Work out the finished part from the listing and answer in its coordinate system (mm). A direction names the side the tool comes from. Coordinates: 2 decimals unless noted, no trailing zeros. Order: outer loops, then holes, each group sorted by start corner. A loop starts at its lowest first (then second) coordinate and runs counter-clockwise, first axis right, second up. Notation, with made-up numbers: M 51,55.25 L 91,55.25 A13 ccw 91,64.25 Z; hole C 46,21.5 d2. An arc over 180 degrees is marked long. Answer in a Markdown table with one row per item. Add a question column.
Item 1: The part is cut by section A-A (y = 1.75). Write down the section's boundary in (x, z), then the cut area to 3 significant figures.
Item 2: The part is cut by section B-B (y = 12). Write down the section's boundary in (x, z).
Item 3: Consider line 1 (X direction, y = 2, z = 6); line 2 (X direction, y = 11, z = 5); line 3 (X direction, y = 14.75, z = 6). Determine where each line is inside the solid, lowest interval first. Write a range as from..to.
Item 4: Which of the six approach directions +Z, -Z, +X, -X, +Y, -Y give full straight-line access (tool end or side, diameter ignored) to faces 1 (the face through (0, 18, 2.25)), 2 (the face through (12.785, 9.486, 4.644)), 3 (the face through (10, 17.5, 6))?
Item 5: Flat-ended cylindrical pins translate along their axes: pin 1 Ø3 at (x, z) = (0, -12) entering from -Y; pin 2 Ø4 at (x, y) = (2.5, 17) entering from +Z; pin 3 Ø4 at (x, z) = (-5, 0.5) entering from -Y. Find the tip coordinate at first contact, or state that the pin passes through.
from build123d import *

# Parameters (mm, degrees)
SKETCH1_R                 = 17
SKETCH1_R_2               = 1.6000000000000005
SKETCH1_R_3               = 1.6000000000000019
SKETCH1_R_4               = 1.5999999999999999
BOSS_EXTRUDE1_DEPTH       = 6.500000000000001
SKETCH2_R                 = 17
SKETCH2_R_2               = 3.4999999999999996
SKETCH2_R_3               = 1.6000000000000012
SKETCH2_R_4               = 1.6000000000000019
SKETCH2_R_5               = 1.5999999999999963
BOSS_EXTRUDE2_DEPTH       = 2
SKETCH3_R                 = 17
SKETCH3_R_2               = 1.2
BOSS_EXTRUDE3_DEPTH       = 2
SKETCH9_R                 = 17
SKETCH9_R_2               = 1.2
SKETCH9_R_3               = 1.5999999999999963
SKETCH9_R_4               = 1.6000000000000012
SKETCH9_R_5               = 1.6000000000000019
BOSS_EXTRUDE6_DEPTH       = 2
BOSS_EXTRUDE4_OUTLINE_R   = 17
BOSS_EXTRUDE4_OUTLINE_R_2 = 1.6
BOSS_EXTRUDE4_DEPTH       = 5
SKETCH10_R                = 17
BOSS_EXTRUDE7_DEPTH       = 4.500000000000001
CHAMFER1_SIZE             = 1.154700538
CHAMFER1_SIZE_2           = 2


# Read off the part's stored shape, not the designer's step: Boss-Extrude4
with BuildPart() as part:
    # Sketch1 → Boss-Extrude1 (new body)
    with BuildSketch(Plane(origin=(0, 0, 0), x_dir=(1, 0, 0), z_dir=(0, 1, 0))):
        with Locations(Location((0, 0, 0), (0, 0, 270))):
            Circle(SKETCH1_R)
        with Locations(Location((0, 12, 0), (0, 0, 270))):
            Circle(SKETCH1_R_2, mode=Mode.SUBTRACT)
        with Locations(Location((10.392304845413268, -5.999999999999997, 0), (0, 0, 270))):
            Circle(SKETCH1_R_3, mode=Mode.SUBTRACT)
        with Locations(Location((-10.39230484541326, -6.000000000000005, 0), (0, 0, 270))):
            Circle(SKETCH1_R_4, mode=Mode.SUBTRACT)
        Polygon((4.04145188432738, -6.999999999999999), (8.082903768654761, -8.7e-16), (4.041451884327381, 6.999999999999999), (-4.041451884327381, 6.999999999999999), (-8.082903768654761, -8.7e-16), (-4.04145188432738, -6.999999999999999), align=None, mode=Mode.SUBTRACT)
    extrude(amount=BOSS_EXTRUDE1_DEPTH)

    # Sketch2 → Boss-Extrude2 (add)
    with BuildSketch(Plane(origin=(0, 6.500000000000001, 0), x_dir=(1, 0, 0), z_dir=(0, 1, 0))):
        with Locations(Location((0, 0, 0), (0, 0, 270))):
            Circle(SKETCH2_R)
        with Locations(Location((0, 0, 0), (0, 0, 270))):
            Circle(SKETCH2_R_2, mode=Mode.SUBTRACT)
        with Locations(Location((0, 12, 0), (0, 0, 270))):
            Circle(SKETCH2_R_3, mode=Mode.SUBTRACT)
        with Locations(Location((10.392304845413268, -5.999999999999997, 0), (0, 0, 270))):
            Circle(SKETCH2_R_4, mode=Mode.SUBTRACT)
        with Locations(Location((-10.39230484541326, -6.000000000000005, 0), (0, 0, 270))):
            Circle(SKETCH2_R_5, mode=Mode.SUBTRACT)
    extrude(amount=BOSS_EXTRUDE2_DEPTH)

    # Sketch3 → Boss-Extrude3 (add)
    with BuildSketch(Plane(origin=(0, 8.5, 0), x_dir=(1, 0, 0), z_dir=(0, 1, 0))):
        with Locations(Location((0, 0, 0), (0, 0, 270))):
            Circle(SKETCH3_R)
        with Locations(Location((0, 0, 0), (0, 0, 270))):
            Circle(SKETCH3_R_2, mode=Mode.SUBTRACT)
        Polygon((3.175426480542944, 11.999999999999996), (1.5877132402714735, 14.75), (-1.5877132402714682, 14.75), (-3.1754264805429417, 11.999999999999995), (-1.5877132402714735, 9.249999999999998), (1.5877132402714729, 9.249999999999998), align=None, mode=Mode.SUBTRACT)
        Polygon((-8.804591605141788, -8.750000000000009), (-7.216878364870316, -6.0000000000000036), (-8.80459160514179, -3.2500000000000013), (-11.980018085684733, -3.250000000000002), (-13.567731325956206, -6.000000000000007), (-11.980018085684732, -8.750000000000009), align=None, mode=Mode.SUBTRACT)
        Polygon((8.804591605141793, -8.75), (11.980018085684742, -8.75), (13.567731325956213, -5.999999999999997), (11.98001808568474, -3.2499999999999925), (8.804591605141791, -3.249999999999992), (7.216878364870319, -5.999999999999996), align=None, mode=Mode.SUBTRACT)
    extrude(amount=BOSS_EXTRUDE3_DEPTH)

    # Sketch9 → Boss-Extrude6 (add)
    with BuildSketch(Plane(origin=(0, 10.5, 0), x_dir=(1, 0, 0), z_dir=(0, 1, 0))):
        with Locations(Location((0, 0, 0), (0, 0, 270))):
            Circle(SKETCH9_R)
        with Locations(Location((0, 0, 0), (0, 0, 270))):
            Circle(SKETCH9_R_2, mode=Mode.SUBTRACT)
        with Locations(Location((-10.39230484541326, -6.000000000000005, 0), (0, 0, 270))):
            Circle(SKETCH9_R_3, mode=Mode.SUBTRACT)
        with Locations(Location((0, 12, 0), (0, 0, 270))):
            Circle(SKETCH9_R_4, mode=Mode.SUBTRACT)
        with Locations(Location((10.392304845413268, -5.999999999999997, 0), (0, 0, 270))):
            Circle(SKETCH9_R_5, mode=Mode.SUBTRACT)
    extrude(amount=BOSS_EXTRUDE6_DEPTH)

    # Boss-Extrude4 outline → Boss-Extrude4 (add)
    with BuildSketch(Plane(origin=(0, 12.5, 0), x_dir=(1, 0, 0), z_dir=(0, 1, 0))):
        Circle(BOSS_EXTRUDE4_OUTLINE_R)
        with Locations((-10.392304845, -6)):
            Circle(BOSS_EXTRUDE4_OUTLINE_R_2, mode=Mode.SUBTRACT)
        with Locations((10.392304845, -6)):
            Circle(BOSS_EXTRUDE4_OUTLINE_R_2, mode=Mode.SUBTRACT)
        with BuildLine():
            Line((-2.34520788, 2.25), (2.34520788, 2.25))
            ThreePointArc((2.34520788, 2.25), (3.25, 0), (2.34520788, -2.25))
            Line((2.34520788, -2.25), (-2.34520788, -2.25))
            ThreePointArc((-2.34520788, -2.25), (-3.25, 0), (-2.34520788, 2.25))
        make_face(mode=Mode.SUBTRACT)
        with Locations((0, 12)):
            Circle(BOSS_EXTRUDE4_OUTLINE_R_2, mode=Mode.SUBTRACT)
    extrude(amount=BOSS_EXTRUDE4_DEPTH)

    # Sketch10 → Boss-Extrude7 (add)
    with BuildSketch(Plane(origin=(0, 17.5, 0), x_dir=(1, 0, 0), z_dir=(0, 1, 0))):
        with Locations(Location((0, 0, 0), (0, 0, 270))):
            Circle(SKETCH10_R)
        with BuildLine():
            Line((-2.345207879911715, -2.2500000000000004), (2.345207879911715, -2.2500000000000004))
            ThreePointArc((2.345207879911715, -2.2500000000000004), (3.2500000000000004, 0), (2.345207879911715, 2.2500000000000004))
            Line((2.345207879911715, 2.2500000000000004), (-2.345207879911715, 2.2500000000000004))
            ThreePointArc((-2.345207879911715, 2.2500000000000004), (-3.2500000000000004, 4e-16), (-2.345207879911715, -2.2500000000000004))
        make_face(mode=Mode.SUBTRACT)
    extrude(amount=BOSS_EXTRUDE7_DEPTH)

    # Sketch5 → Cut-Revolve2 (revolve, cut)
    with BuildSketch(Plane(origin=(0, 0, 0), x_dir=(0, 0, -1), z_dir=(1, 0, 0)), mode=Mode.PRIVATE) as cut_revolve2_sk:
        Polygon((-17, 18.535898384862204), (-15.000000000000002, 22), (-17, 22.000000000000004), align=None)
    revolve(cut_revolve2_sk.sketch.rotate(Axis((0, 0, 0), (0, 1, 0)), 180), axis=Axis((0, 0, 0), (0, 1, 0)), mode=Mode.SUBTRACT)

    # Chamfer1
    # the kernel refuses this chamfer: 2, 1.154700538 mm, written as the material it adds along each edge
    with BuildSketch(Plane(origin=(-2.2883428e-10, 12.5, 0), x_dir=(-0.7079171545098687, 0, -0.706295478076032), z_dir=(-0.706295478076032, 0, 0.7079171545098687))) as chamfer1_piece_1:
        Polygon((3.2500000002288263 - CHAMFER1_SIZE, 0), (3.2500000002288343, -CHAMFER1_SIZE_2), (3.2500000002288263, 0), align=None)
    revolve(axis=Axis((-2.2883428e-10, 12.5, 0), (0, -1, 0)), revolution_arc=270.1314019865591)
    with BuildSketch(Plane(origin=(-7.519379389291984, 12.5, -2.2500000000000004), x_dir=(0, 0.9998132206222079, -0.01932676561270072), z_dir=(1, 0, 0))) as chamfer1_piece_2_section:
        Polygon((CHAMFER1_SIZE_2 * 0.999813220622, CHAMFER1_SIZE_2 * 0.0193267656127), (-CHAMFER1_SIZE * 0.019326765619, CHAMFER1_SIZE * 0.999813220951), (0, 0), align=None)
    chamfer1_piece_2 = extrude(amount=15.038758778583968, mode=Mode.PRIVATE)
    chamfer1_piece_2 = chamfer1_piece_2 - Plane(origin=(0, 13.182227685151497, 0), x_dir=(-1.8e-16, 0, 1), z_dir=(0, -1, 0)) * Cylinder(1.2, 39, mode=Mode.PRIVATE)
    add(chamfer1_piece_2)
    with BuildSketch(Plane(origin=(2.2883428e-10, 12.5, 0), x_dir=(0.7079171545098687, 0, 0.706295478076032), z_dir=(0.706295478076032, 0, -0.7079171545098687))) as chamfer1_piece_3:
        Polygon((3.2500000002288343, -CHAMFER1_SIZE_2), (3.250000000228834 - CHAMFER1_SIZE, 0), (3.250000000228834, 0), align=None)
    revolve(axis=Axis((2.2883428e-10, 12.5, 0), (0, -1, 0)), revolution_arc=270.1314019865591)
    with BuildSketch(Plane(origin=(7.519379389291984, 12.5, 2.2500000000000004), x_dir=(0, 0.9998132206222079, 0.01932676561270072), z_dir=(-1, 0, 0))) as chamfer1_piece_4_section:
        Polygon((CHAMFER1_SIZE_2 * 0.999813220622, CHAMFER1_SIZE_2 * 0.0193267656127), (-CHAMFER1_SIZE * 0.019326765619, CHAMFER1_SIZE * 0.999813220951), (0, 0), align=None)
    chamfer1_piece_4 = extrude(amount=15.038758778583968, mode=Mode.PRIVATE)
    chamfer1_piece_4 = chamfer1_piece_4 - Plane(origin=(0, 13.182227685146668, 0), x_dir=(-1.8e-16, 0, 1), z_dir=(0, -1, 0)) * Cylinder(1.2, 39, mode=Mode.PRIVATE)
    add(chamfer1_piece_4)


solid = part.part
Reply:
| question | item | result |
|---|---|---|
| 1 | outline | C 0,0 d34; hole C -10.39,6 d3.2; hole M -8.08,0 L -4.04,-7 L 4.04,-7 L 8.08,0 L 4.04,7 L -4.04,7 Z; hole C 0,-12 d3.2; hole C 10.39,6 d3.2 |
| 1 | area | 714 mm2 |
| 2 | outline | C 0,0 d34; hole C -10.39,6 d3.2; hole C 0,-12 d3.2; hole C 0,0 d2.4; hole C 10.39,6 d3.2 |
| 3 | line 1 | x = -15.91..-11.99, -8.79..-4.62, 4.62..8.79, 11.99..15.91 |
| 3 | line 2 | x = -16.25..-11.64, -9.14..9.14, 11.64..16.25 |
| 3 | line 3 | x = -15.91..-11.99, -8.79..8.79, 11.99..15.91 |
| 4 | face 1 | +Y |
| 4 | face 2 | none |
| 4 | face 3 | -Y |
| 5 | pin 1 | stops at y = 17.5 |
| 5 | pin 2 | stops at z = 16.99 |
| 5 | pin 3 | stops at y = 6.5 |
